Build history of the part. All positions in model axes, mm. A direction names the side the tool comes from. Round coordinates to 2 decimals unless told otherwise and drop trailing zeros. Write each loop counter-clockwise with the first axis right and the second up, starting at its lowest first coordinate (ties: lowest second). Pieces come first, ordered by that corner, then holes.
from build123d import *

# Parameters (mm, degrees)
SKETCH1_W           = 60
SKETCH1_H           = 50
BOSS_EXTRUDE1_DEPTH = 2
BOSS_EXTRUDE2_DEPTH = 13
SKETCH3_W           = 9
SKETCH3_H           = 15
BOSS_EXTRUDE3_DEPTH = 1.75
FILLET1_R           = 1.5
CUT_EXTRUDE1_REACH  = 81.53
SKETCH4_R           = 2.005
SKETCH5_W           = 1
SKETCH5_H           = 51.75
BOSS_EXTRUDE4_DEPTH = 20
SKETCH6_W           = 54
SKETCH6_H           = 2
CUT_EXTRUDE2_DEPTH  = 47
BOSS_EXTRUDE5_REACH = 86.57


with BuildPart() as part:
    # Sketch1 → Boss-Extrude1 (new body)
    with BuildSketch(Plane(origin=(0, 0, 0), x_dir=(1, 0, 0), z_dir=(0, 1, 0))):
        with Locations((30, 25)):
            Rectangle(SKETCH1_W, SKETCH1_H)
    extrude(amount=BOSS_EXTRUDE1_DEPTH)

    # Sketch2 → Boss-Extrude2 (add)
    with BuildSketch(Plane(origin=(0, 2, 0), x_dir=(1, 0, 0), z_dir=(0, 1, 0))):
        Polygon((60, 0), (60, 50), (0, 50), (0, 0), (3, 0), (3, 47), (57, 47), (57, 0), align=None)
    extrude(amount=BOSS_EXTRUDE2_DEPTH)

    # Sketch3 → Boss-Extrude3 (add)
    with BuildSketch(Plane(origin=(0, 0, -50), x_dir=(-1, 0, 0), z_dir=(0, 0, -1))):
        with Locations((-55.5, 7.5)):
            Rectangle(SKETCH3_W, SKETCH3_H)
    extrude(amount=BOSS_EXTRUDE3_DEPTH)

    # Fillet1
    fillet1_edges = [part.edges().sort_by_distance(p)[0] for p in [
        (51, 7.5, -50),
    ]]
    fillet(fillet1_edges, radius=FILLET1_R)

    # Sketch4 → Cut-Extrude1 (cut, up to next)
    with BuildSketch(Plane(origin=(0, 0, -50), x_dir=(-1, 0, 0), z_dir=(0, 0, -1)), mode=Mode.PRIVATE) as cut_extrude1_sk1:
        with Locations((-45, 5.6)):
            Circle(SKETCH4_R)
    cut_extrude1_tool1 = extrude(cut_extrude1_sk1.sketch, amount=-CUT_EXTRUDE1_REACH, mode=Mode.PRIVATE) & part.part
    # Sketch4 → Cut-Extrude1 (cut, up to next)
    with BuildSketch(Plane(origin=(0, 0, -50), x_dir=(-1, 0, 0), z_dir=(0, 0, -1)), mode=Mode.PRIVATE) as cut_extrude1_sk2:
        with Locations((-35, 5.6)):
            Circle(SKETCH4_R)
    cut_extrude1_tool2 = extrude(cut_extrude1_sk2.sketch, amount=-CUT_EXTRUDE1_REACH, mode=Mode.PRIVATE) & part.part
    # Sketch4 → Cut-Extrude1 (cut, up to next)
    with BuildSketch(Plane(origin=(0, 0, -50), x_dir=(-1, 0, 0), z_dir=(0, 0, -1)), mode=Mode.PRIVATE) as cut_extrude1_sk3:
        with Locations((-25, 5.6)):
            Circle(SKETCH4_R)
    cut_extrude1_tool3 = extrude(cut_extrude1_sk3.sketch, amount=-CUT_EXTRUDE1_REACH, mode=Mode.PRIVATE) & part.part
    # Sketch4 → Cut-Extrude1 (cut, up to next)
    with BuildSketch(Plane(origin=(0, 0, -50), x_dir=(-1, 0, 0), z_dir=(0, 0, -1)), mode=Mode.PRIVATE) as cut_extrude1_sk4:
        with Locations((-15, 5.6)):
            Circle(SKETCH4_R)
    cut_extrude1_tool4 = extrude(cut_extrude1_sk4.sketch, amount=-CUT_EXTRUDE1_REACH, mode=Mode.PRIVATE) & part.part
    add(cut_extrude1_tool1.solids().sort_by_distance((45, 5.6, -50))[0], mode=Mode.SUBTRACT)
    add(cut_extrude1_tool2.solids().sort_by_distance((35, 5.6, -50))[0], mode=Mode.SUBTRACT)
    add(cut_extrude1_tool3.solids().sort_by_distance((25, 5.6, -50))[0], mode=Mode.SUBTRACT)
    add(cut_extrude1_tool4.solids().sort_by_distance((15, 5.6, -50))[0], mode=Mode.SUBTRACT)

    # Sketch5 → Boss-Extrude4 (add)
    with BuildSketch(Plane(origin=(0, 15, 0), x_dir=(1, 0, 0), z_dir=(0, 1, 0))):
        with Locations((59.5, 25.875)):
            Rectangle(SKETCH5_W, SKETCH5_H)
    extrude(amount=BOSS_EXTRUDE4_DEPTH)

    # Sketch6 → Cut-Extrude2 (cut)
    with BuildSketch(Plane.XY):
        with Locations((30, 1)):
            Rectangle(SKETCH6_W, SKETCH6_H)
    extrude(amount=-CUT_EXTRUDE2_DEPTH, mode=Mode.SUBTRACT)

    # Sketch7 → Boss-Extrude5 (add, up to next)
    with BuildSketch(Plane(origin=(3, 0, 0), x_dir=(0, 0, -1), z_dir=(1, 0, 0)), mode=Mode.PRIVATE) as boss_extrude5_sk1:
        Polygon((0, 2), (0, 0), (2, 0), (47, 13), (47, 15), align=None)
    boss_extrude5_tool1 = extrude(boss_extrude5_sk1.sketch, amount=BOSS_EXTRUDE5_REACH, mode=Mode.PRIVATE) - part.part
    add(boss_extrude5_tool1.solids().sort_by_distance((3, 7.115265, -22.629283))[0])


solid = part.part
1) Pin check, flat tips, straight feed: pin 1 Ø6 at (y, z) = (25.5, -34.5) entering from -X; pin 2 Ø12 at (x, y) = (24.5, 10) entering from -Z; pin 3 Ø1.5 at (x, z) = (53, -44.5) entering from +Y. Stop position of each tip, or through.
Results:
pin 1: stops at x = 59
pin 2: stops at z = -50
pin 3: stops at y = 14.52
2) Slice it at A-A (x = 15). Write the cut outline in (y, z) (3 decimals), plus the area to 3 significant figures.
Results:
outline: (0, -50) - (3.595, -50) - (3.595, -47) - (0, -47) - close; (0, -2) - (13, -47) - (7.605, -47) - (7.605, -50) - (15, -50) - (15, -47) - (2, 0) - (0, 0) - close
area: 140 mm2
3) Mould opens along X. For faces 4 (the flat face through (60, 17, -26)), 5 (the flat face through (3, 4, -34)), 6 (the flat face through (30, 0, -49)), 7 (the cylindrical face through (50.55, 7.6, -50.43)) say: released by +X, released by -X, zero draft, split by the parting line, or undercut.
Results:
face 4: released by +X
face 5: undercut
face 6: zero draft
face 7: released by -X
4) Slice it at B-B (y = 5.6). Count the separate pieces of the cut face and the enclosed holes in it, plus the area to 3 significant figures.
Results:
separate pieces: 4
enclosed holes: 0
area: 882 mm2
5) Which spindle directions (+Z, -Z, +X, -X, +Y, -Y) get a long thin tool onto all of the face, cutting with end or side? Do faces 1 (the flat face through (25, 9, -50)), 2 (the flat face through (29.622, 6.409, -24.185)), 3 (the flat face through (32, 15, -49)). Say none if no direction does.
Results:
face 1: -Z, -X, +Y, -Y
face 2: -Y
face 3: +Z, -Z, -X, +Y
6) Slice it at C-C (x = 6). Write the cut outline in (y, z), plus the area to 3 significant figures.
Results:
outline: (0, -50) - (15, -50) - (15, -47) - (2, 0) - (0, 0) - (0, -2) - (13, -47) - (0, -47) - close
area: 152 mm2
7) Wall check: L1, parallel to X at y = 12, z = -10.5; L2, parallel to Y at x = 35, z = -48.75 (3 decimals); L3, parallel to X at y = 17.5, z = -21. Give the ranges that are in metal, low to high.
Results:
L1: x = 0 to 3, 57 to 60
L2: y = 0 to 3.595, 7.605 to 15
L3: x = 59 to 60
8) Slice it at D-D (y = 11.5). Write the cut outline in (x, z), plus the area to 3 significant figures.
Results:
outline: (0, -50) - (49.5, -50) arc R1.5 cw to (51, -51.5) - (51, -51.75) - (60, -51.75) - (60, 0) - (57, 0) - (57, -34.35) - (3, -34.35) - (3, 0) - (0, 0) - close; hole (3, -47) - (57, -47) - (57, -41.81) - (3, -41.81) - close
area: 881 mm2
